```python
from build123d import *

# Parameters (mm, degrees)
SKETCH_1_W               = 440
SKETCH_1_H               = 107
SM_BASE_FLANGE_1_DEPTH   = 5
SKETCH_8_R               = 22.5
CUT_EXTRUDE_1_DEPTH      = 10
SKETCH_9_R               = 3
CUT_EXTRUDE_2_DEPTH      = 10
SKETCH_10_R              = 16.5
CUT_EXTRUDE_3_DEPTH      = 10
SKETCH_11_R              = 4
CUT_EXTRUDE_4_DEPTH      = 10
SKETCH_12_R              = 3
CUT_EXTRUDE_5_DEPTH      = 10
MIRROR_3_COPY_1_SKETCH_R = 3
MIRROR_3_COPY_1_DEPTH    = 10
FILLET_1_R               = 1
SKETCH_13_R              = 1.5
CUT_EXTRUDE_6_DEPTH      = 10


# Sheet-metal steps are written as plain solids
with BuildPart() as part:
    # Sketch 1 → 基体-法兰1 (new body)
    with BuildSketch(Plane.XY):
        Rectangle(SKETCH_1_W, SKETCH_1_H)
    extrude(amount=-SM_BASE_FLANGE_1_DEPTH)

    # 草图8 → 切除-拉伸1 (cut)
    with BuildSketch(Plane.XY):
        with Locations((175, 8.5)):
            Circle(SKETCH_8_R)
    cut_extrude_1 = extrude(amount=-CUT_EXTRUDE_1_DEPTH, mode=Mode.SUBTRACT)

    # 草图9 → 切除-拉伸2 (cut)
    with BuildSketch(Plane.XY):
        with Locations((175, 41)):
            Circle(SKETCH_9_R)
        with Locations((207.5, 8.5)):
            Circle(SKETCH_9_R)
        with Locations((175, -24)):
            Circle(SKETCH_9_R)
        with Locations((142.5, 8.5)):
            Circle(SKETCH_9_R)
    cut_extrude_2 = extrude(amount=-CUT_EXTRUDE_2_DEPTH, mode=Mode.SUBTRACT)

    # 镜向1: 切除-拉伸1, 切除-拉伸2 across plane
    add(cut_extrude_1.mirror(Plane(origin=(0, 0, 0), x_dir=(0, 0, 1), z_dir=(1, 0, 0))), mode=Mode.SUBTRACT)
    add(cut_extrude_2.mirror(Plane(origin=(0, 0, 0), x_dir=(0, 0, 1), z_dir=(1, 0, 0))), mode=Mode.SUBTRACT)

    # 草图10 → 切除-拉伸3 (cut)
    with BuildSketch(Plane(origin=(0, 0, -5), x_dir=(-1, 0, 0), z_dir=(0, 0, -1))):
        with Locations((105, 8.5)):
            Circle(SKETCH_10_R)
    extrude(amount=-CUT_EXTRUDE_3_DEPTH, mode=Mode.SUBTRACT)

    # 草图11 → 切除-拉伸4 (cut)
    with BuildSketch(Plane(origin=(0, 0, -5), x_dir=(-1, 0, 0), z_dir=(0, 0, -1))):
        with Locations((0, -5.630506542)):
            Circle(SKETCH_11_R)
    extrude(amount=-CUT_EXTRUDE_4_DEPTH, mode=Mode.SUBTRACT)

    # 草图12 → 切除-拉伸5 (cut)
    with BuildSketch(Plane(origin=(0, 0, -5), x_dir=(-1, 0, 0), z_dir=(0, 0, -1))):
        with Locations((-70, 33.5)):
            Circle(SKETCH_12_R)
        with Locations((-50, 33.5)):
            Circle(SKETCH_12_R)
    cut_extrude_5 = extrude(amount=-CUT_EXTRUDE_5_DEPTH, mode=Mode.SUBTRACT)

    # 镜向2: 切除-拉伸5 across plane
    add(cut_extrude_5.mirror(Plane(origin=(0, 0, 0), x_dir=(0, 0, 1), z_dir=(1, 0, 0))), mode=Mode.SUBTRACT)

    # 镜向3: 切除-拉伸5 across plane
    add(cut_extrude_5.mirror(Plane.ZX.offset(8.5)), mode=Mode.SUBTRACT)

    # 镜向3 copy 1 sketch → 镜向3 copy 1 (cut)
    with BuildSketch(Plane(origin=(0, 17, -5), x_dir=(1, 0, 0), z_dir=(0, 0, -1))):
        with Locations((-70, 33.5)):
            Circle(MIRROR_3_COPY_1_SKETCH_R)
        with Locations((-50, 33.5)):
            Circle(MIRROR_3_COPY_1_SKETCH_R)
    extrude(amount=-MIRROR_3_COPY_1_DEPTH, mode=Mode.SUBTRACT)

    # 圆角1
    fillet_1_edges = [part.edges().sort_by_distance(p)[0] for p in [
        (220, -53.5, -2.5),
        (-220, -53.5, -2.5),
        (-220, 53.5, -2.5),
        (220, 53.5, -2.5),
    ]]
    fillet(fillet_1_edges, radius=FILLET_1_R)

    # 草图13 → 切除-拉伸6 (cut)
    with BuildSketch(Plane(origin=(0, 0, -5), x_dir=(-1, 0, 0), z_dir=(0, 0, -1))):
        with Locations((-100, 41.75)):
            Circle(SKETCH_13_R)
        with Locations((-90, 41.75)):
            Circle(SKETCH_13_R)
        with Locations((-90, 34.75)):
            Circle(SKETCH_13_R)
        with Locations((-100, 34.75)):
            Circle(SKETCH_13_R)
    extrude(amount=-CUT_EXTRUDE_6_DEPTH, mode=Mode.SUBTRACT)


solid = part.part
```
For this review, take the finished solid that the model builds, in its own axes (mm). Round coordinates to 2 decimals unless told otherwise and drop trailing zeros. Loops run counter-clockwise (first coordinate to the right, second up) from the corner with the lowest first, then second, coordinate; pieces in that order, holes last.
Q1. Mouldability with a two-part tool opening along X and no side actions: class faces 1 (the face through (196.46, 15.26, -2.46)), 2 (the face through (-88.516, 9.225, -2.535)), 3 (the face through (-3, 1, 0)) as +X half, -X half, draft (parallel to the pull), parting line (faces both ways), or undercut.
Result sheet:
face 1: undercut
face 2: undercut
face 3: draft
Q2. Add section C-C on x = 0. Write out the cut boundary in (y, z).
Result sheet:
outline: (-53.5, -5) - (-9.63, -5) - (-9.63, 0) - (-53.5, 0) - close; (-1.63, -5) - (53.5, -5) - (53.5, 0) - (-1.63, 0) - close
Q3. Add section B-B on z = -3.65. Give the number of separate pieces and of enclosed holes in the cut face, plus the area to 3 significant figures.
Result sheet:
separate pieces: 1
enclosed holes: 24
area: 42,500 mm2
Q4. Add section A-A on x = -105. Write out the cut boundary in (y, z).
Result sheet:
outline: (-53.5, -5) - (-8, -5) - (-8, 0) - (-53.5, 0) - close; (25, -5) - (53.5, -5) - (53.5, 0) - (25, 0) - close
Q5. To check wall thickness, follow line 1 along X through (y, z) = (-17, -3.5); line 2 along Y through (x, z) = (50, -2.8); line 3 along Y through (x, z) = (175, -1). State the ranges of each line that lie inside material, in increasing order.
Result sheet:
line 1: x = -220 to -72.96, -67.04 to -52.96, -47.04 to 47.04, 52.96 to 67.04, 72.96 to 220
line 2: y = -53.5 to -19.5, -13.5 to 30.5, 36.5 to 53.5
line 3: y = -53.5 to -27, -21 to -14, 31 to 38, 44 to 53.5
